Verification items for this drawing (mm, ordinates from the low corner). A direction names the side the tool comes from. Coordinates: 2 decimals unless noted, no trailing zeros. Write each loop counter-clockwise with the first axis right and the second up, starting at its lowest first coordinate (ties: lowest second). Pieces come first, ordered by that corner, then holes. Notation, with made-up numbers: (69.5, -23) -> (76.5, -23) arc R14 cw to (76.5, 3) -> close; hole circle Ø10 at (21.5, 87). An arc over 180 degrees is marked (long way). Use CSV: the item, a comma, the result in double quotes.
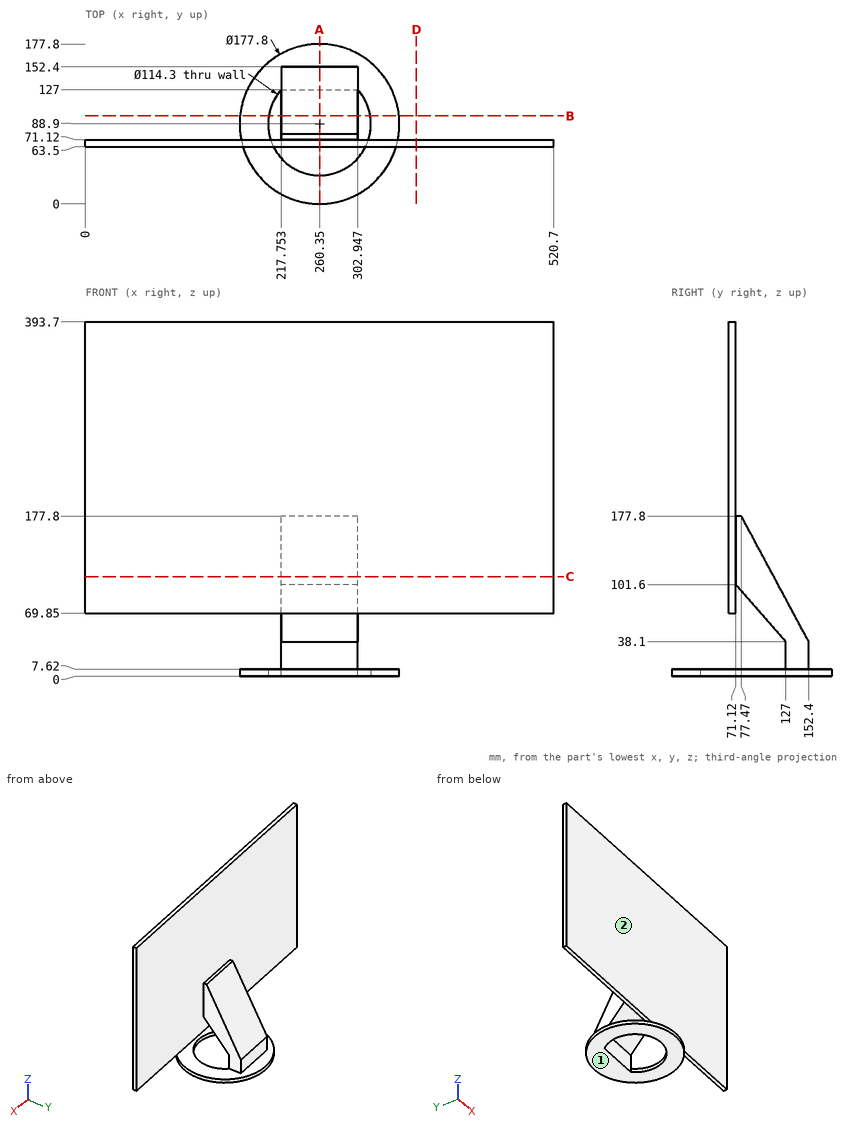
1) Cross-section at C-C (z = 110.5). Record the boundary of the cut face in (x, y), plus the area to 3 significant figures.
Return value:
outline,"(0, 63.5) -> (520.7, 63.5) -> (520.7, 71.12) -> (302.95, 71.12) -> (302.95, 113.57) -> (217.75, 113.57) -> (217.75, 71.12) -> (0, 71.12) -> close"
area,"7,580 mm2"
2) Cross-section at D-D (x = 368). Record the boundary of the cut face in (y, z), plus the area to 3 significant figures.
Return value:
outline,"(63.5, 69.85) -> (71.12, 69.85) -> (71.12, 393.7) -> (63.5, 393.7) -> close"
area,"2,470 mm2"
3) Scan lines: L1, parallel to Y at x = 260.35, z = 5.5; L2, parallel to X at y = 88, z = 3; L3, parallel to Z at x = 233, y = 23.5. Record each from-to range of solid material in increasing order.
Return value:
L1,"0 to 31.75, 127 to 177.8"
L2,"171.45 to 203.21, 317.49 to 349.25"
L3,"0 to 7.62"
4) Cross-section at B-B (y = 98). Record the boundary of the cut face in (x, z).
Return value:
outline,"(171.92, 0) -> (203.93, 0) -> (203.93, 7.62) -> (171.92, 7.62) -> close; (217.75, 71.05) -> (302.95, 71.05) -> (302.95, 139.52) -> (217.75, 139.52) -> close; (316.77, 0) -> (348.78, 0) -> (348.78, 7.62) -> (316.77, 7.62) -> close"
5) Cross-section at A-A (x = 260.35). Record the boundary of the cut face in (y, z).
Return value:
outline,"(0, 0) -> (31.75, 0) -> (31.75, 7.62) -> (0, 7.62) -> close; (63.5, 69.85) -> (71.12, 69.85) -> (71.12, 101.6) -> (127, 38.1) -> (127, 0) -> (177.8, 0) -> (177.8, 7.62) -> (152.4, 7.62) -> (152.4, 38.1) -> (77.47, 177.8) -> (71.12, 177.8) -> (71.12, 393.7) -> (63.5, 393.7) -> close"
6) Set-up check for the marked faces 1 and 2: record each of +Z, -Z, +X, -X, +Y, -Y from which the full face is reachable in a straight line by a thin tool's end or side.
Return value:
face 1,"-Z, +X, -X, +Y, -Y"
face 2,"+Z, +X, -X, -Y"
7) Gauge pin test, flat ends, axial feed: pin 1 (8 mm diameter, centred on x = 181, z = 341.5, fed in from -Y); pin 2 (24.5 mm diameter, centred on y = 115.5, z = 72.5, fed in from -X); pin 3 (8 mm diameter, centred on x = 258, z = 64, fed in from +Y). Record the tip position at first contact, or that the pin passes through.
Return value:
pin 1,"y = 63.5"
pin 2,"x = 217.75"
pin 3,"y = 140.65"
